Part model, mm, in its own coordinate system. A direction names the side the tool comes from. Coordinates: 2 decimals unless noted, no trailing zeros. Order: outer loops, then holes, each group sorted by start corner. A loop starts at its lowest first (then second) coordinate and runs counter-clockwise, first axis right, second up. Notation, with made-up numbers: M 32.5,48.25 L 53.5,48.25 A24 ccw 53.5,80.25 Z; hole C 48.5,63.25 d1. An arc over 180 degrees is marked long. Write item = value, one per line. Start each with the question number.
from build123d import *

# Parameters (mm, degrees)
SKETCH_1_R          = 12
EXTRUDE_1_DEPTH     = 9.5
SKETCH_2_R          = 7
EXTRUDE_2_DEPTH     = 42.5
SKETCH_3_R          = 9
EXTRUDE_3_DEPTH     = 10.3
SKETCH_4_R          = 13
EXTRUDE_4_DEPTH     = 9.8
CUT_EXTRUDE_START   = -10
CUT_EXTRUDE_3_DEPTH = 10
CHAMFER_1_SIZE      = 1


with BuildPart() as part:
    # 草圖1 → 伸長1 (new body)
    with BuildSketch(Plane(origin=(0, 0, 0), x_dir=(0, 0, -1), z_dir=(1, 0, 0))):
        Circle(SKETCH_1_R)
    extrude(amount=EXTRUDE_1_DEPTH)

    # 草圖2 → 伸長2 (add)
    with BuildSketch(Plane(origin=(9.5, 0, 0), x_dir=(0, 0, -1), z_dir=(1, 0, 0))):
        Circle(SKETCH_2_R)
    extrude(amount=EXTRUDE_2_DEPTH)

    # 草圖3 → 伸長3 (add)
    with BuildSketch(Plane.ZY):
        with Locations(Location((0, 0, 0), (0, 0, 180))):
            Circle(SKETCH_3_R)
    extrude(amount=EXTRUDE_3_DEPTH)

    # 草圖4 → 伸長4 (add)
    with BuildSketch(Plane.ZY.offset(10.3)):
        Circle(SKETCH_4_R)
    extrude(amount=EXTRUDE_4_DEPTH)

    # 草圖5 → 除料-伸長3 (cut)
    with BuildSketch(Plane(origin=(9.5, 0, 0), x_dir=(0, 0, -1), z_dir=(1, 0, 0)).offset(CUT_EXTRUDE_START)):
        with BuildLine():
            Line((-11, 4.795831523), (-11, -4.795831523))
            ThreePointArc((-11, -4.795831523), (-12, 0), (-11, 4.795831523))
        make_face()
        with BuildLine():
            Line((11, 4.795831523), (11, -4.795831523))
            ThreePointArc((11, -4.795831523), (12, 0), (11, 4.795831523))
        make_face()
    extrude(amount=CUT_EXTRUDE_3_DEPTH, mode=Mode.SUBTRACT)

    # 導角1
    chamfer_1_edges = [part.edges().sort_by_distance(p)[0] for p in [
        (-20.1, 0, -13),
        (-10.3, 0, -13),
        (9.5, 12, 0),
        (9.5, -12, 0),
        (0, 12, 0),
        (0, -12, 0),
        (52, 0, 7),
    ]]
    chamfer(chamfer_1_edges, length=CHAMFER_1_SIZE - 0.0001)  # a hair under: the kernel refuses the full size


solid = part.part
Item 1: Pull direction X, two halves, no side cores. Call faces 1 (the conical face through (9.3, 11.2, -0.2)), 2 (the cylindrical face through (5, 12, 0)), 3 (the conical face through (0.2, -11.2, 0.2)): pulls with the +X half, pulls with the -X half, needs draft (parallel to the pull), parting line crosses it, or undercut.
Item 2: Cut at A-A, the plane z = 0. Write the cut outline in (x, y), and give its area (3 significant figures).
Item 3: Cut at B-B, the plane x = 29. Write the cut outline in (y, z).
Item 4: 3-axis set-ups, long thin cutter, end or side, ignore diameter. For faces 4 (the conical face through (0.2, 11.2, -0.2)), 5 (the flat face through (5, 0, 11)), 6 (the cylindrical face through (5, -12, 0)), 7 (the cylindrical face through (29.96, -2.681, -6.466)), 8 (the cylindrical face through (-5.078, -6.083, 6.633)): which of +Z, -Z, +X, -X, +Y, -Y reach the whole face in a straight line?
Item 5: Cut at C-C, the plane x = -3.5. Write the cut outline in (y, z), and give its area (3 significant figures).
Item 6: Wall check: line 1 along X through (y, z) = (-7, 8.25); line 2 along X through (y, z) = (3.25, 6.5); line 3 along X through (y, z) = (-11, -3.75). Give the ranges that are in metal, low to high. Write a range as [from, to].
Item 7: Flat gauge pins, fed straight in: pin 1 (4 mm diameter, centred on y = -8, z = -3, fed in from +X); pin 2 (1 mm diameter, centred on x = 30.5, y = 0.5, fed in from -Z); pin 3 (7.5 mm diameter, centred on x = 4, y = 1, fed in from +Z); pin 4 (1.5 mm diameter, centred on x = 26, z = -9, fed in from -Y). Where does each tip first touch, or does it go through?
Filled sheet:
q1.face_1 = pulls with the +X half
q1.face_2 = needs draft
q1.face_3 = undercut
q2.outline = M -20.1,-12 L -19.1,-13 L -11.3,-13 L -10.3,-12 L -10.3,-9 L 0,-9 L 0,-11 L 1,-12 L 8.5,-12 L 9.5,-11 L 9.5,-7 L 51,-7 L 52,-6 L 52,6 L 51,7 L 9.5,7 L 9.5,11 L 8.5,12 L 1,12 L 0,11 L 0,9 L -10.3,9 L -10.3,12 L -11.3,13 L -19.1,13 L -20.1,12 Z
q2.area = 1,260 mm2
q3.outline = C 0,0 d14
q4.face_4 = +Y
q4.face_5 = +Z, +X, +Y, -Y
q4.face_6 = +X, -Y
q4.face_7 = +X
q4.face_8 = none
q5.outline = C 0,0 d18
q5.area = 254 mm2
q6.line_1 = [-20.1, -10.3], [0, 9.5]
q6.line_2 = [-20.1, 9.5]
q6.line_3 = [-20.1, -10.3], [0.62, 8.88]
q7.pin_1 = 51.46
q7.pin_2 = -7
q7.pin_3 = 11
q7.pin_4 = through
